```python
from build123d import *

# Parameters (mm, degrees)
SKETCH1_R           = 70
BOSS_EXTRUDE1_DEPTH = 15
SKETCH2_R           = 5
CUT_EXTRUDE1_DEPTH  = 15
SKETCH3_R           = 2.5
CUT_EXTRUDE2_DEPTH  = 16


with BuildPart() as part:
    # Sketch1 → Boss-Extrude1 (new body)
    with BuildSketch(Plane(origin=(0, 0, 0), x_dir=(1, 0, 0), z_dir=(0, 1, 0))):
        Circle(SKETCH1_R)
    extrude(amount=BOSS_EXTRUDE1_DEPTH)

    # Sketch2 → Cut-Extrude1 (cut)
    with BuildSketch(Plane(origin=(0, 15, 0), x_dir=(1, 0, 0), z_dir=(0, 1, 0))):
        Circle(SKETCH2_R)
    extrude(amount=-CUT_EXTRUDE1_DEPTH, mode=Mode.SUBTRACT)

    # Sketch3 → Cut-Extrude2 (cut, through all)
    with BuildSketch(Plane.XZ):
        with Locations((0, 23)):
            Circle(SKETCH3_R)
        with Locations((19.918584287, -11.5)):
            Circle(SKETCH3_R)
        with Locations((-19.918584287, -11.5)):
            Circle(SKETCH3_R)
    extrude(amount=-CUT_EXTRUDE2_DEPTH, mode=Mode.SUBTRACT)


solid = part.part
```
Could you check a few things on this model? Use its own coordinates, in mm. Coordinates: 2 decimals unless noted, no trailing zeros. Write each loop counter-clockwise with the first axis right and the second up, starting at its lowest first coordinate (ties: lowest second). Pieces come first, ordered by that corner, then holes. Notation, with made-up numbers: (11.5, -18) - (64.5, -18) arc R13 ccw to (64.5, 2) - close; hole circle Ø9 at (-32.5, -18.5). An arc over 180 degrees is marked (long way). Use a Markdown table: item, result.
Q1. Imagine slicing it at A-A (z = 0). List the corners of the cut face in (x, y) for me, and give its area (3 significant figures).
Geometry check:
| item | result |
|---|---|
| outline | (-70, 0) - (-5, 0) - (-5, 15) - (-70, 15) - close; (5, 0) - (70, 0) - (70, 15) - (5, 15) - close |
| area | 1,950 mm2 |
Q2. I'm going to push flat-ended pins straight in: pin 1 Ø3 at (y, z) = (7.5, -46.5) entering from -X; pin 2 Ø4 at (x, y) = (-45.5, 1.5) entering from -Z; pin 3 Ø1.5 at (x, y) = (-50.5, 8) entering from -Z. Where does each tip first touch, or does it pass through?
Geometry check:
| item | result |
|---|---|
| pin 1 | stops at x = -53.62 |
| pin 2 | stops at z = -54.84 |
| pin 3 | stops at z = -49.24 |
Q3. Please list where these lines run through material, in increasing order: L1, parallel to Z at x = 0, y = 10.75; L2, parallel to Z at x = -4, y = 10.5; L3, parallel to Z at x = -16, y = 11.5.
Geometry check:
| item | result |
|---|---|
| L1 | z = -70 to -5, 5 to 20.5, 25.5 to 70 |
| L2 | z = -69.89 to -3, 3 to 69.89 |
| L3 | z = -68.15 to 68.15 |
Q4. Thinking about a two-plate mould opening in X: for faces 1 (the flat face through (-1, 15, 15)), 2 (the cylindrical face through (-0.33, 7.4, 25.48)), 3 (the cylindrical face through (17.935, 7.395, -13.021)), 4 (the cylindrical face through (-55.55, 7.395, 42.594)), which applies, +X half, -X half, draft (parallel to the pull), parting line (faces both ways), or undercut?
Geometry check:
| item | result |
|---|---|
| face 1 | draft |
| face 2 | undercut |
| face 3 | undercut |
| face 4 | parting line |
Q5. Imagine slicing it at D-D (z = 23). List the corners of the cut face in (x, y) for me.
Geometry check:
| item | result |
|---|---|
| outline | (-66.11, 0) - (-2.5, 0) - (-2.5, 15) - (-66.11, 15) - close; (2.5, 0) - (66.11, 0) - (66.11, 15) - (2.5, 15) - close |
Q6. Imagine slicing it at C-C (y = 10). List the corners of the cut face in (x, z) for me.
Geometry check:
| item | result |
|---|---|
| outline | circle Ø140 at (0, 0); hole circle Ø5 at (-19.92, -11.5); hole circle Ø10 at (0, 0); hole circle Ø5 at (0, 23); hole circle Ø5 at (19.92, -11.5) |
Q7. Imagine slicing it at B-B (x = 0). List the corners of the cut face in (y, z) for me, and give its area (4 significant figures).
Geometry check:
| item | result |
|---|---|
| outline | (0, -70) - (15, -70) - (15, -5) - (0, -5) - close; (0, 5) - (15, 5) - (15, 20.5) - (0, 20.5) - close; (0, 25.5) - (15, 25.5) - (15, 70) - (0, 70) - close |
| area | 1,875 mm2 |
